Source: CAD feature listing. Evaluate the final solid. Frame: model axes, mm. A direction names the side the tool comes from. Coordinates: 2 decimals unless noted, no trailing zeros. Loops run counter-clockwise (first coordinate to the right, second up) from the corner with the lowest first, then second, coordinate; pieces in that order, holes last. Notation, with made-up numbers: (-17.5, 15.25) -> (11.5, 15.25) arc R13 cw to (11.5, 23.25) -> close; hole circle Ø2 at (-28, 76). An arc over 180 degrees is marked (long way). Answer as CSV lines item,"result".
from build123d import *

# Parameters (mm, degrees)
SKETCH1_W                                           = 30
SKETCH1_H                                           = 20
BOSS_EXTRUDE1_DEPTH                                 = 50
CUT_EXTRUDE5_DEPTH                                  = 56.901917603
CUT_EXTRUDE2_DEPTH                                  = 20
SKETCH6_W                                           = 6
SKETCH6_H                                           = 22
CUT_EXTRUDE3_DEPTH                                  = 5
SKETCH7_R                                           = 1.75
CUT_EXTRUDE4_DEPTH                                  = 55.298200385
CBORE_FOR_M3_HEX_SOCKET_HEAD_CAP_SCREW1_D           = 3.4
CBORE_FOR_M3_HEX_SOCKET_HEAD_CAP_SCREW1_CBORE_D     = 7
CBORE_FOR_M3_HEX_SOCKET_HEAD_CAP_SCREW1_CBORE_DEPTH = 38.4
FILLET1_START                                       = -6
FILLET1_DEPTH                                       = 22


with BuildPart() as part:
    # Sketch1 → Boss-Extrude1 (new body)
    with BuildSketch(Plane.XY):
        with Locations((-0.000813035, 4.942227855)):
            Rectangle(SKETCH1_W, SKETCH1_H)
    extrude(amount=BOSS_EXTRUDE1_DEPTH)

    # Sketch3 → Cut-Extrude5 (cut, through all)
    with BuildSketch(Plane(origin=(0, 14.942227855, 0), x_dir=(1, 0, 0), z_dir=(0, 1, 0))):
        with BuildLine():
            Line((-4.500783142, -24.000000003), (-4.500176076, -40))
            ThreePointArc((-4.500176076, -40), (-0.000631376, -44.4995447), (4.498913324, -40))
            Line((4.498913324, -40), (4.498913324, -24.000000003))
            ThreePointArc((4.498913324, -24.000000003), (-0.000934909, -19.50015177), (-4.500783142, -24.000000003))
        make_face()
    extrude(amount=-CUT_EXTRUDE5_DEPTH, mode=Mode.SUBTRACT)

    # Sketch5 → Cut-Extrude2 (cut)
    with BuildSketch(Plane(origin=(0, 14.942227855, 0), x_dir=(1, 0, 0), z_dir=(0, 1, 0))):
        with BuildLine():
            Line((-9.751131515, -40), (-9.751131515, -24.000000003))
            ThreePointArc((-9.751131515, -24.000000003), (-8.000813035, -22.249681523), (-6.250494556, -24.000000003))
            Line((-6.250494556, -24.000000003), (-6.250494556, -40))
            ThreePointArc((-6.250494556, -40), (-8.000813035, -41.75031848), (-9.751131515, -40))
        make_face()
    cut_extrude2 = extrude(amount=-CUT_EXTRUDE2_DEPTH, mode=Mode.SUBTRACT)

    # Sketch6 → Cut-Extrude3 (cut)
    with BuildSketch(Plane.XZ.offset(5.057772145)):
        with Locations((-8.000813035, 32.000000001)):
            Rectangle(SKETCH6_W, SKETCH6_H)
    cut_extrude3 = extrude(amount=-CUT_EXTRUDE3_DEPTH, mode=Mode.SUBTRACT)

    # Sketch7 → Cut-Extrude4 (cut, through all)
    with BuildSketch(Plane.XY.offset(50)):
        with Locations((-11.000813035, 4.942227855)):
            Circle(SKETCH7_R)
    cut_extrude4 = extrude(amount=-CUT_EXTRUDE4_DEPTH, mode=Mode.SUBTRACT)

    # CBORE for M3 Hex Socket Head Cap Screw1 (through all)
    with Locations(Plane.XY.offset(50)):
        with Locations((-11.000813035, 4.942227855)):
            cbore_for_m3_hex_socket_head_cap_screw1 = CounterBoreHole(CBORE_FOR_M3_HEX_SOCKET_HEAD_CAP_SCREW1_D / 2, CBORE_FOR_M3_HEX_SOCKET_HEAD_CAP_SCREW1_CBORE_D / 2, CBORE_FOR_M3_HEX_SOCKET_HEAD_CAP_SCREW1_CBORE_DEPTH)

    # Fillet1: read off the stored shape, not the designer's step
    # Fillet1 outline → Fillet1 (cut)
    with BuildSketch(Plane(origin=(0, 0, 0), x_dir=(1, 0, 0), z_dir=(0, 1, 0)).offset(FILLET1_START)):
        with BuildLine():
            ThreePointArc((14.999186965, -40), (12.070254777, -47.071067812), (4.999186965, -50))
            Line((4.999186965, -50), (14.999186965, -50))
            Line((14.999186965, -50), (14.999186965, -40))
        make_face()
        with BuildLine():
            Line((-15.000813035, -50), (-5.000813035, -50))
            ThreePointArc((-5.000813035, -50), (-12.071880847, -47.071067812), (-15.000813035, -40))
            Line((-15.000813035, -40), (-15.000813035, -50))
        make_face()
    extrude(amount=FILLET1_DEPTH, mode=Mode.SUBTRACT)

    # Mirror1: Cut-Extrude2, Cut-Extrude3, Cut-Extrude4, CBORE for M3 Hex Socket Head Cap Screw1 across plane
    add(cut_extrude2.mirror(Plane(origin=(-0.000813035, 0, 0), x_dir=(0, 0, 1), z_dir=(1, 0, 0))), mode=Mode.SUBTRACT)
    add(cut_extrude3.mirror(Plane(origin=(-0.000813035, 0, 0), x_dir=(0, 0, 1), z_dir=(1, 0, 0))), mode=Mode.SUBTRACT)
    add(cut_extrude4.mirror(Plane(origin=(-0.000813035, 0, 0), x_dir=(0, 0, 1), z_dir=(1, 0, 0))), mode=Mode.SUBTRACT)
    add(cbore_for_m3_hex_socket_head_cap_screw1.mirror(Plane(origin=(-0.000813035, 0, 0), x_dir=(0, 0, 1), z_dir=(1, 0, 0))), mode=Mode.SUBTRACT)


solid = part.part
(1) Cut plane A-A (y = 10). Return the cut outline in (x, z), then the cut area to 3 significant figures.
Computed values:
outline,"(-15, 0) -> (15, 0) -> (15, 40) arc R10 ccw to (5, 50) -> (-5, 50) arc R10 ccw to (-15, 40) -> close; hole (-9.75, 24) arc R1.75 ccw to (-6.25, 24) -> (-6.25, 40) arc R1.75 ccw to (-9.75, 40) -> close; hole (-4.5, 24) arc R4.5 ccw to (4.5, 24) -> (4.5, 40) arc R4.5 ccw to (-4.5, 40) -> close; hole (6.25, 24) arc R1.75 ccw to (9.75, 24) -> (9.75, 40) arc R1.75 ccw to (6.25, 40) -> close"
area,"1,120 mm^2"
(2) Cut plane D-D (y = -3.5). Return the cut outline in (x, z).
Computed values:
outline,"(-15, 0) -> (15, 0) -> (15, 40) arc R10 ccw to (5, 50) -> (-5, 50) arc R10 ccw to (-15, 40) -> close; hole (-11, 21) -> (-5, 21) -> (-5, 43) -> (-11, 43) -> close; hole (-4.5, 24) arc R4.5 ccw to (4.5, 24) -> (4.5, 40) arc R4.5 ccw to (-4.5, 40) -> close; hole (5, 21) -> (11, 21) -> (11, 43) -> (5, 43) -> close"
(3) Access query for faces 1 (the flat face through (8, -3, 21)), 2 (the cylindrical face through (0.1, 5.1, 19.5)), 3 (the flat face through (-15.001, 5, 20)), 4 (the cylindrical face through (-14.497, 5.096, 30.908)). Directions: +Z, -Z, +X, -X, +Y, -Y. A direction counts if a zero-diameter tool reaches every point of the face in a straight line with its end or side. Return the directions, or none.
Computed values:
face 1,"-Y"
face 2,"+Y, -Y"
face 3,"+Z, -Z, -X, +Y, -Y"
face 4,"+Z"
(4) Draft query along X for faces 5 (the cylindrical face through (-14.017, 2.58, 44.326)), 6 (the flat face through (-9.751, 12, 32)), 7 (the cylindrical face through (-7.366, 7.547, 41.631)), 8 (the flat face through (14.999, 5, 20)). Return one class per face: released by +X, released by -X, zero draft, split by the parting line, or undercut.
Computed values:
face 5,"released by -X"
face 6,"undercut"
face 7,"undercut"
face 8,"released by +X"
(5) Material intervals for L1, parallel to X at y = 10.75, z = 38; L2, parallel to X at y = 2.5, z = 23; L3, parallel to X at y = 5.25, z = 16, sorted ascending. Write a range as [from, to].
Computed values:
L1,"[-15, -9.75], [-6.25, -4.5], [4.5, 6.25], [9.75, 15]"
L2,"[-15, -13.51], [-6.56, -4.39], [4.39, 6.56], [13.51, 15]"
L3,"[-15, -14.49], [-7.51, 7.51], [14.49, 15]"
(6) Cut plane B-B (x = 10.5). Return the cut outline in (y, z), then the cut area to 3 significant figures.
Computed values:
outline,"(-5.06, 0) -> (3.26, 0) -> (3.26, 11.6) -> (1.48, 11.6) -> (1.48, 48.35) -> (-5.06, 48.35) -> (-5.06, 43) -> (-0.06, 43) -> (-0.06, 21) -> (-5.06, 21) -> close; (6.62, 0) -> (14.94, 0) -> (14.94, 48.35) -> (8.41, 48.35) -> (8.41, 11.6) -> (6.62, 11.6) -> close"
area,"563 mm^2"
(7) Cut plane C-C (z = 29). Return the cut outline in (x, y), then the cut area to 3 significant figures.
Computed values:
outline,"(-15, -5.06) -> (-11, -5.06) -> (-11, -0.06) -> (-9.75, -0.06) -> (-9.75, 1.67) arc R3.5 cw (long way) to (-9.75, 8.21) -> (-9.75, 14.94) -> (-15, 14.94) -> close; (-6.25, -0.06) -> (-5, -0.06) -> (-5, -5.06) -> (-4.5, -5.06) -> (-4.5, 14.94) -> (-6.25, 14.94) -> close; (4.5, -5.06) -> (5, -5.06) -> (5, -0.06) -> (6.25, -0.06) -> (6.25, 14.94) -> (4.5, 14.94) -> close; (9.75, -0.06) -> (11, -0.06) -> (11, -5.06) -> (15, -5.06) -> (15, 14.94) -> (9.75, 14.94) -> (9.75, 8.21) arc R3.5 cw (long way) to (9.75, 1.67) -> close"
area,"199 mm^2"
(8) Pin query (flat end, axial travel): pin 1 Ø7.5 at (x, y) = (12, 5) entering from +Z; pin 2 Ø1.8 at (x, z) = (-9.5, 34) entering from -Y; pin 3 Ø3.5 at (x, y) = (-9.5, 3.5) entering from +Z. Return the tip coordinate at first contact, or that it passes through.
Computed values:
pin 1,"z = 48.42"
pin 2,"y = -0.06"
pin 3,"z = 49.61"
